Work out the finished part from the listing and answer in its coordinate system (mm). Round coordinates to 2 decimals unless told otherwise and drop trailing zeros. Order: outer loops, then holes, each group sorted by start corner. A loop starts at its lowest first (then second) coordinate and runs counter-clockwise, first axis right, second up. Notation, with made-up numbers: (-21, 22.5) - (19, 22.5) arc R26 cw to (19, 44.5) - close; hole circle Ø5 at (60.5, -16.5). An arc over 180 degrees is marked (long way). Put each result on its own line as item: value.
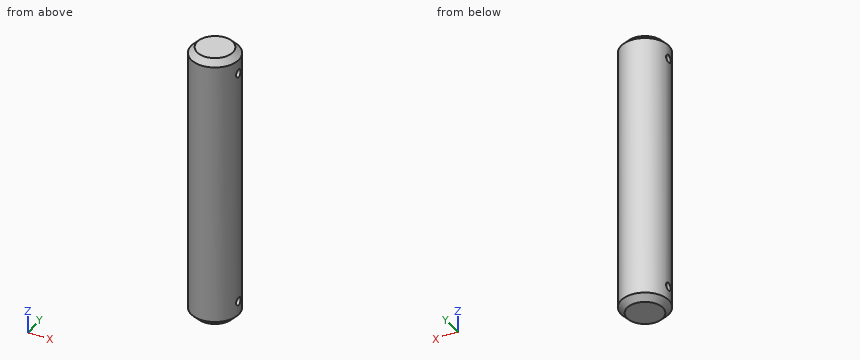
```python
from build123d import *

# Parameters (mm, degrees)
CUT_EXTRUDE1_DEPTH      = 37.013886211
CUT_EXTRUDE1_DEPTH_BACK = 37.013886211
SKETCH2_R               = 1


with BuildPart() as part:
    # Sketch1 → Revolve1 (revolve)
    with BuildSketch(Plane(origin=(0, 0, 0), x_dir=(0, 0, -1), z_dir=(1, 0, 0)), mode=Mode.PRIVATE) as revolve1_sk:
        Polygon((35, 0), (35, 4.5), (33.5, 6), (-33.5, 6), (-35, 4.5), (-35, 0), align=None)
    revolve(revolve1_sk.sketch.rotate(Axis((0, 0, 35), (0, 0, -1)), 90), axis=Axis((0, 0, 35), (0, 0, -1)))

    # Sketch2 → Cut-Extrude1 (cut, two sides: drawn at the far end of the back side and taken through both)
    with BuildSketch(Plane(origin=(0, 0, 0), x_dir=(0, 0, -1), z_dir=(1, 0, 0)).offset(-CUT_EXTRUDE1_DEPTH_BACK)):
        with Locations((30, 0)):
            Circle(SKETCH2_R)
        with Locations((-30, 0)):
            Circle(SKETCH2_R)
    extrude(amount=CUT_EXTRUDE1_DEPTH + CUT_EXTRUDE1_DEPTH_BACK, mode=Mode.SUBTRACT)


solid = part.part
```
1) Given pin 1 Ø2.5 at (y, z) = (0, 30) entering from +X; pin 2 Ø4 at (y, z) = (-4, -7) entering from -X; pin 3 Ø3 at (x, y) = (-4.5, -4.5) entering from +Z; pin 4 Ø4 at (y, z) = (-3, 14) entering from -X, each flat-ended and moving along its own axis, determine where each tip first touches the part or whether it passes through.
Findings below:
pin 1: stops at x = 6
pin 2: stops at x = -5.66
pin 3: stops at z = 34.64
pin 4: stops at x = -5.92
2) A cutting plane is placed at B-B on z = 30. Write down the section's boundary in (x, y), then the cut area to 3 significant figures.
Findings below:
outline: (-5.92, -1) arc R6 ccw to (5.92, -1) - close; (-5.92, 1) - (5.92, 1) arc R6 ccw to start
area: 89.2 mm2
3) Straight lines are drawn through the part: L1, parallel to Z at x = 0.25, y = 0; L2, parallel to Y at x = -2.5, z = 30; L3, parallel to Y at x = -1, z = -30. For each, find the intervals that lie inside material, in ascending order. Write a range as from..to.
Findings below:
L1: z = -35..-31, -29..29, 31..35
L2: y = -5.45..-1, 1..5.45
L3: y = -5.92..-1, 1..5.92
4) A cutting plane is placed at C-C on x = 3.75. Give the number of separate pieces and of enclosed holes in the cut face, then the cut area to 3 significant figures.
Findings below:
separate pieces: 1
enclosed holes: 2
area: 643 mm2
5) A cutting plane is placed at D-D on z = -21. Write down the section's boundary in (x, y).
Findings below:
outline: circle Ø12 at (0, 0)
6) A cutting plane is placed at A-A on y = 0. Write down the section's boundary in (x, z).
Findings below:
outline: (-6, -33.5) - (-4.5, -35) - (4.5, -35) - (6, -33.5) - (6, -31) - (-6, -31) - close; (-6, -29) - (6, -29) - (6, 29) - (-6, 29) - close; (-6, 31) - (6, 31) - (6, 33.5) - (4.5, 35) - (-4.5, 35) - (-6, 33.5) - close
